Geometry: final body of the model. Coordinates: model frame, mm. A direction names the side the tool comes from. Give positions to 0.01 mm unless a question says otherwise; leave off trailing zeros. Loops run counter-clockwise (first coordinate to the right, second up) from the corner with the lowest first, then second, coordinate; pieces in that order, holes last. Notation, with made-up numbers: M 85.5,75 L 123.5,75 A26 cw 123.5,89 Z; hole C 20,70.25 d11. An arc over 180 degrees is marked long. Put each result on its own line as item: value.
```python
from build123d import *

# Parameters (mm, degrees)
SKETCH1_R           = 4.9
BOSS_EXTRUDE1_DEPTH = 5
SKETCH2_R           = 7.5
BOSS_EXTRUDE2_DEPTH = 2
SKETCH3_R           = 5.9
BOSS_EXTRUDE3_DEPTH = 8
CHAMFER1_SIZE       = 1


with BuildPart() as part:
    # Sketch1 → Boss-Extrude1 (new body)
    with BuildSketch(Plane(origin=(0, 0, 0), x_dir=(1, 0, 0), z_dir=(0, 1, 0))):
        with Locations(Location((0, 0, 0), (0, 0, 270))):
            Circle(SKETCH1_R)
    extrude(amount=BOSS_EXTRUDE1_DEPTH)

    # Sketch2 → Boss-Extrude2 (add)
    with BuildSketch(Plane(origin=(0, 1.999999904, 0), x_dir=(1, 0, 0), z_dir=(0, 1, 0))):
        with Locations(Location((0, 0, 0), (0, 0, 270))):
            Circle(SKETCH2_R)
    extrude(amount=-BOSS_EXTRUDE2_DEPTH)

    # Sketch3 → Boss-Extrude3 (add)
    with BuildSketch(Plane(origin=(0, 0, 0), x_dir=(1, 0, 0), z_dir=(0, 1, 0))):
        with Locations(Location((0, 0, 0), (0, 0, 270))):
            Circle(SKETCH3_R)
    extrude(amount=-BOSS_EXTRUDE3_DEPTH)

    # Chamfer1
    chamfer1_edges = [part.edges().sort_by_distance(p)[0] for p in [
        (0, -8, -5.9),
    ]]
    chamfer(chamfer1_edges, length=CHAMFER1_SIZE)


solid = part.part
```
Item 1: Section B-B on z = 0. Output: boundary loops of the cut face in (x, y).
Output values:
outline: M -7.5,0 L -5.9,0 L -5.9,-7 L -4.9,-8 L 4.9,-8 L 5.9,-7 L 5.9,0 L 7.5,0 L 7.5,2 L 4.9,2 L 4.9,5 L -4.9,5 L -4.9,2 L -7.5,2 Z
Item 2: Section A-A on x = 0. Output: boundary loops of the cut face in (y, z), then the cut area to 3 significant figures.
Output values:
outline: M -8,-4.9 L -7,-5.9 L 0,-5.9 L 0,-7.5 L 2,-7.5 L 2,-4.9 L 5,-4.9 L 5,4.9 L 2,4.9 L 2,7.5 L 0,7.5 L 0,5.9 L -7,5.9 L -8,4.9 Z
area: 153 mm²
Item 3: Section C-C on y = -5.75. Output: boundary loops of the cut face in (x, z), then the cut area to 3 significant figures.
Output values:
outline: C 0,0 d11.8
area: 109 mm²
Item 4: Pin query (flat end, axial travel): pin 1 Ø5 at (y, z) = (3.5, -1.5) entering from -X; pin 2 Ø3 at (x, y) = (-5, 2.5) entering from +Z; pin 3 Ø3 at (x, y) = (4, -2.5) entering from -Z; pin 4 Ø4 at (y, z) = (1, 2.5) entering from +X. Return the tip coordinate at first contact, or that it passes through.
Output values:
pin 1: x = -7.5
pin 2: z = 6.59
pin 3: z = -5.34
pin 4: x = 7.48
Item 5: Line query: probe 1 along Y at (x, z) = (-5.5, 2.25); probe 2 along X at (y, z) = (-5.5, 0); probe 3 along Z at (x, y) = (-4, 3.5). Output: solid intervals per line, ascending. Write a range as [from, to].
Output values:
probe 1: [0, 2]
probe 2: [-5.9, 5.9]
probe 3: [-2.83, 2.83]
Item 6: Section D-D on y = 0.5. Output: boundary loops of the cut face in (x, z), then the cut area to 3 significant figures.
Output values:
outline: C 0,0 d15
area: 177 mm²
Item 7: Set-up query: faces 1 (the cylindrical face through (-5.76, -3.45, -1.28)), 2 (the flat face through (0, 5, 0)), 3 (the cylindrical face through (1.472, 3.479, 4.674)). Return all of +Z, -Z, +X, -X, +Y, -Y with unobstructed straight access to the full face (end or side cutting, diameter ignored); none if empty.
Output values:
face 1: -Y
face 2: +Z, -Z, +X, -X, +Y
face 3: +Y
